Read the model definition and answer for the solid it produces. Units are mm, in the model's axes. A direction names the side the tool comes from. Give positions to 0.01 mm unless a question says otherwise; leave off trailing zeros. Order: outer loops, then holes, each group sorted by start corner. A loop starts at its lowest first (then second) coordinate and runs counter-clockwise, first axis right, second up. Notation, with made-up numbers: (-11.75, -7) - (47.25, -7) arc R10 ccw to (47.25, 5) - close; hole circle Ø6 at (74, 60). An arc over 180 degrees is marked (long way). Write each question's results on one line, items separated by ' | '.
from build123d import *

# Parameters (mm, degrees)
F1_DEPTH = 19.05
F3_DEPTH = 12.7


with BuildPart() as f1:
    # F0 (on Front) → F1 (new body)
    with BuildSketch(Plane.XZ):
        with BuildLine():
            Line((114.3, 149.934994), (0, 149.934994))
            Line((0, 149.934994), (-114.3, 149.934994))
            Line((-114.3, 149.934994), (-222.022257, -116.581239))
            Line((-222.022257, -116.581239), (-114.3, -116.581239))
            ThreePointArc((-114.3, -116.581239), (0, 1.407281), (114.3, -116.581239))
            Line((114.3, -116.581239), (222.022257, -116.581239))
            Line((222.022257, -116.581239), (114.3, 149.934994))
        make_face()
    extrude(amount=F1_DEPTH)

    # F2 (on Front) → F3 (cut)
    with BuildSketch(Plane.XZ):
        Polygon((-9.652, 24.14524), (0, 24.14524), (9.652, 24.14524), (9.652, 151.098922), (0, 151.098922), (-9.652, 151.098922), align=None)
    extrude(amount=F3_DEPTH, mode=Mode.SUBTRACT)


solid = f1.part
(1) The mould has two halves that part along X. Classify faces 3 (the face through (168.915, -9.392, 14.811)), 4 (the face through (2, -14, 149.935)), 5 (the face through (0, -12.7, 88)): pulls with the +X half, pulls with the -X half, needs draft (parallel to the pull), parting line crosses it, or undercut.
Conclusion:
face 3: pulls with the +X half | face 4: needs draft | face 5: undercut
(2) Each of these flat-tipped pins is pushed along its axis until it touches: pin 1 (6 mm diameter, centred on x = 1.5, z = 105, fed in from +Y); pin 2 (10 mm diameter, centred on y = -7.5, z = 108.5, fed in from -X); pin 3 (6.5 mm diameter, centred on y = -4.5, z = 107, fed in from +X). Where does it stop, or does it pass through?
Conclusion:
pin 1: y = -12.7 | pin 2: x = -133.07 | pin 3: x = 132.97
(3) Section B-B (y = -16) is taken. Give the vertices of the cut face in (x, z) (3 decimals), plus the area to 3 significant figures.
Conclusion:
outline: (-222.022, -116.581) - (-114.3, -116.581) arc R114.358 cw (long way) to (114.3, -116.581) - (222.022, -116.581) - (114.3, 149.935) - (-114.3, 149.935) - close | area: 68,300 mm^2
(4) Section C-C (x = 0) is taken. Give the vertices of the cut face in (y, z) (3 decimals), plus the area to 3 significant figures.
Conclusion:
outline: (-19.05, 1.407) - (0, 1.407) - (0, 24.145) - (-12.7, 24.145) - (-12.7, 149.935) - (-19.05, 149.935) - close | area: 1,230 mm^2
(5) Consider probe 1 along X at (y, z) = (-6.5, -101.5); probe 2 along X at (y, z) = (-8.5, -85.5); probe 3 along Z at (x, y) = (66.5, -17.25) (3 decimals). Determine where each line is inside the solid, lowest interval first. Write a range as [from, to].
Conclusion:
probe 1: [-215.93, -113.78], [113.78, 215.93] | probe 2: [-209.46, -111.01], [111.01, 209.46] | probe 3: [-19.916, 149.935]
(6) Section D-D (z = 116.5) is taken. Give the vertices of the cut face in (x, y).
Conclusion:
outline: (-127.81, -19.05) - (127.81, -19.05) - (127.81, 0) - (9.65, 0) - (9.65, -12.7) - (-9.65, -12.7) - (-9.65, 0) - (-127.81, 0) - close
(7) For faces 1 (the face through (-9.652, -6, 88)), 2 (the face through (167, -9, -116.581)), determine the directions among +Z, -Z, +X, -X, +Y, -Y from which every point of the face is accessible in a straight line to the end or side of a thin tool.
Conclusion:
face 1: +Z, +Y | face 2: -Z, +X, -X, +Y, -Y
(8) Section A-A (z = -64) is taken. Give the vertices of the cut face in (x, y), plus the area to 3 significant figures.
Conclusion:
outline: (-200.77, -19.05) - (-103.35, -19.05) - (-103.35, 0) - (-200.77, 0) - close; (103.35, -19.05) - (200.77, -19.05) - (200.77, 0) - (103.35, 0) - close | area: 3,710 mm^2
